from build123d import *

# Parameters (mm, degrees)
SKETCH1_W                                     = 76.2
SKETCH1_H                                     = 44.45
BOSS_EXTRUDE1_DEPTH                           = 7.1501
CUT_EXTRUDE1_DEPTH                            = 80.696389849
CBORE_FOR_1_4_SOCKET_HEAD_CAP_SCREW1_AT_COUNT = 2
CBORE_FOR_1_4_SOCKET_HEAD_CAP_SCREW1_AT_PITCH = 50.8
CAVITY1_START                                 = -11.732042998
CAVITY1_OUTLINE_W                             = 78.1
CAVITY1_OUTLINE_H                             = 25
CAVITY1_DEPTH                                 = 2.228722608


# Read off the part's stored shape, not the designer's step: Cavity1
with BuildPart() as part:
    # Sketch1 → Boss-Extrude1 (new, symmetric)
    with BuildSketch(Plane.XY):
        Rectangle(SKETCH1_W, SKETCH1_H)
    extrude(amount=BOSS_EXTRUDE1_DEPTH, both=True)

    # Sketch2 → Cut-Extrude1 (cut, through all)
    with BuildSketch(Plane(origin=(38.1, 0, 0), x_dir=(0, 0, -1), z_dir=(1, 0, 0))):
        Polygon((7.1501, -6.343018915), (-7.1501, -22.225), (7.1501, -22.225), align=None)
        Polygon((-7.1501, 22.225), (7.1501, 6.343018915), (7.1501, 22.225), align=None)
    extrude(amount=-CUT_EXTRUDE1_DEPTH, mode=Mode.SUBTRACT)

    # Sketch6 → CBORE for 1/4 Socket Head Cap Screw1 (revolve, cut)
    with BuildSketch(Plane(origin=(-25.4, 0, 7.1501), x_dir=(0, -1, 0), z_dir=(1, 0, 0))):
        Polygon((0, 0), (0, 14.3002), (4.0132, 14.3002), (3.3782, 13.6652), (3.3782, 6.35), (5.55625, 6.35), (5.55625, 0.635), (6.19125, 0), align=None)
    cbore_for_1_4_socket_head_cap_screw1 = revolve(axis=Axis((-25.4, 0, 13.5001), (0, 0, -1)), mode=Mode.SUBTRACT)

    # CBORE for 1/4 Socket Head Cap Screw1 at: CBORE for 1/4 Socket Head Cap Screw1 ×2
    with Locations(*[(i * CBORE_FOR_1_4_SOCKET_HEAD_CAP_SCREW1_AT_PITCH, 0, 0) for i in range(1, CBORE_FOR_1_4_SOCKET_HEAD_CAP_SCREW1_AT_COUNT)]):
        add(cbore_for_1_4_socket_head_cap_screw1, mode=Mode.SUBTRACT)

    # Sketch8 → 7/16 (0.4375) Diameter Hole1 (revolve, cut)
    with BuildSketch(Plane(origin=(0, 0, 7.1501), x_dir=(0, -1, 0), z_dir=(1, 0, 0))):
        Polygon((0, 0), (0, 14.3002), (6.19125, 14.3002), (5.55625, 13.6652), (5.55625, 0.635), (6.19125, 0), align=None)
    revolve(axis=Axis((0, 0, 13.5001), (0, 0, -1)), mode=Mode.SUBTRACT)

    # Cavity1 outline → Cavity1 (cut)
    with BuildSketch(Plane(origin=(0, 0, 0), x_dir=(1, 0, 0), z_dir=(0, 0.7431448254773938, 0.6691306063588588)).offset(CAVITY1_START)):
        with Locations((-0.95, -9.5)):
            Rectangle(CAVITY1_OUTLINE_W, CAVITY1_OUTLINE_H)
    extrude(amount=CAVITY1_DEPTH, mode=Mode.SUBTRACT)


solid = part.part
Design review of the part built by this model. Coordinates are the model's own, in mm. A direction names the side the tool comes from. Coordinates: 2 decimals unless noted, no trailing zeros. Loops run counter-clockwise (first coordinate to the right, second up) from the corner with the lowest first, then second, coordinate; pieces in that order, holes last. Notation, with made-up numbers: M -22,68.25 L 18,68.25 A27 ccw 18,87.25 Z; hole C 16,32 d10. An arc over 180 degrees is marked long. Use one line per item in the form item = value.
(1) Clearance check with flat-ended pins moving along their axes: P1, Ø10, axis at x = 5, y = 11.5, coming from the -Z side; P2, Ø3, axis at x = 5, z = 2, coming from the -Y side; P3, Ø3.5, axis at x = 24, y = -2, coming from the +Z side. State where each tip first meets the part, or that it passes through.
Return value:
P1 = -7.01
P2 = -15.94
P3 = 0.8
(2) Consider section C-C (y = 0). Give the number of separate pieces and of enclosed holes in the cut face, and give its area (3 significant figures).
Return value:
separate_pieces = 4
enclosed_holes = 0
area = 680 mm2
(3) Draft analysis for pull direction X (two halves, no side actions). For faces 3 (the face through (28.7, 0.73, -2.81)), 4 (the face through (-0.5, -12.7, -0.1)), 5 (the face through (38.1, 1, 2)), state which applies: pulls with the +X half, pulls with the -X half, needs draft (parallel to the pull), parting line crosses it, or undercut.
Return value:
face_3 = undercut
face_4 = needs draft
face_5 = pulls with the +X half
(4) Consider section B-B (z = -3). Write out the cut boundary in (x, y), and give its area (3 significant figures).
Return value:
outline = M -38.1,-10.09 L 38.1,-10.09 L 38.1,10.95 L -38.1,10.95 Z; hole C -25.4,0 d6.76; hole C 0,0 d11.11; hole C 25.4,0 d6.76
area = 1,430 mm2
(5) Consider section A-A (x = 0). Write out the cut boundary in (y, z) (3 decimals), and give its area (3 significant figures).
Return value:
outline = M -19.226,7.15 L -6.38,-7.117 L -6.343,-7.15 L -6.191,-7.15 L -5.556,-6.515 L -5.556,6.515 L -6.191,7.15 Z; M 5.556,-6.515 L 6.191,-7.15 L 6.343,-7.15 L 22.225,7.15 L 6.191,7.15 L 5.556,6.515 Z
area = 227 mm2
(6) For line 1 along X through (y, z) = (0, -3.25); line 2 along X through (y, z) = (0, 2.8); line 3 along Z through (x, y) = (6, -13.5), list the stretches that pass through material, from the lowest coordinate up. Write a range as from..to.
Return value:
line_1 = -38.1..-28.78, -22.02..-5.56, 5.56..22.02, 28.78..38.1
line_2 = -38.1..-30.96, -19.84..-5.56, 5.56..19.84, 30.96..38.1
line_3 = 0.79..7.15
(7) For faces 1 (the face through (30.824, 1.204, 3.698)), 2 (the face through (-38.1, 1, 2)), list the 3-axis set-ups (+Z, -Z, +X, -X, +Y, -Y) from which the entire face can be reached by the end or side of a thin tool; tool diameter is ignored.
Return value:
face_1 = +Z
face_2 = +Z, -Z, -X, +Y, -Y
(8) Consider section D-D (x = -25.4). Write out the cut boundary in (y, z) (3 decimals).
Return value:
outline = M -19.226,7.15 L -6.38,-7.117 L -6.343,-7.15 L -4.013,-7.15 L -3.378,-6.515 L -3.378,0.8 L -5.556,0.8 L -5.556,6.515 L -6.191,7.15 Z; M 3.378,-6.515 L 4.013,-7.15 L 6.343,-7.15 L 22.225,7.15 L 6.191,7.15 L 5.556,6.515 L 5.556,0.8 L 3.378,0.8 Z
